from build123d import *

# Parameters (mm, degrees)
SKETCH1_R           = 381
SKETCH1_R_2         = 279.4
BOSS_EXTRUDE1_DEPTH = 19.05
CIRPATTERN1_COUNT   = 24


with BuildPart() as part:
    # Sketch1 → Boss-Extrude1 (new body)
    with BuildSketch(Plane(origin=(0, 0, 0), x_dir=(1, 0, 0), z_dir=(0, 1, 0))):
        Circle(SKETCH1_R)
        Circle(SKETCH1_R_2, mode=Mode.SUBTRACT)
    extrude(amount=BOSS_EXTRUDE1_DEPTH)

    # Sketch2 → 1 (1) Diameter Hole1 (revolve, cut)
    with BuildSketch(Plane(origin=(0, 19.05, -330.2), x_dir=(0, 0, 1), z_dir=(1, 0, 0))):
        Polygon((0, 0), (0, 39.630929862), (12.7, 32), (12.7, 0), align=None)
    f_1_1_diameter_hole1 = revolve(axis=Axis((0, 25.4, -330.2), (0, -1, 0)), mode=Mode.SUBTRACT)

    # CirPattern1: 1 (1) Diameter Hole1 ×24 about axis
    cirpattern1_axis = Axis((0, 0, 0), (0, 1, 0))
    for i in range(1, CIRPATTERN1_COUNT):
        add(f_1_1_diameter_hole1.rotate(cirpattern1_axis, i * 360 / CIRPATTERN1_COUNT), mode=Mode.SUBTRACT)


solid = part.part
Could you check a few things on this model? Use its own coordinates, in mm. Give positions to 0.01 mm unless a question says otherwise; leave off trailing zeros. Order: outer loops, then holes, each group sorted by start corner. A loop starts at its lowest first (then second) coordinate and runs counter-clockwise, first axis right, second up. Notation, with made-up numbers: (-11, 4) -> (10, 4) arc R21 cw to (10, 17) -> close; hole circle Ø7 at (70.5, 35.25). An arc over 180 degrees is marked (long way). Answer in a Markdown table with one row per item. Add a question column.
Item 1: We'd pull the mould along Z, two halves only. Please class faces 1 (the cylindrical face through (-302.35, 9.39, 231.83)), 2 (the flat face through (-115, 0, -256)), 3 (the cylindrical face through (273.37, 9.66, 163.45)): pulls with the +Z half, pulls with the -Z half, needs draft (parallel to the pull), parting line crosses it, or undercut.
Item 2: Imagine slicing it at C-C (y = 5.75). Count the separate pieces of the cut face and the enclosed holes in it, and give its area (3 significant figures).
Item 3: Imagine slicing it at A-A (z = -121.5). List the corners of the cut face in (x, y) for me, and give its area (3 significant figures).
Item 4: I'm going to push flat-ended pins straight in: P1, Ø6, axis at x = 59.5, y = 15.5, coming from the +Z side; P2, Ø2, axis at y = 13.5, z = 23.5, coming from the -X side; P3, Ø2, axis at y = 9.5, z = -265.5, coming from the +X side. Where does each tip first touch, or does it pass through?
Item 5: Please list where these lines run through material, in increasing order: probe 1 along Z at (x, y) = (0, 6.75); probe 2 along X at (y, z) = (6.5, 165.1); probe 3 along Z at (x, y) = (288, 9).
Item 6: Imagine slicing it at B-B (x = -43). List the corners of the cut face in (y, z) for me, and give its area (3 significant figures).
Result:
| question | item | result |
|---|---|---|
| 1 | face 1 | parting line crosses it |
| 1 | face 2 | needs draft |
| 1 | face 3 | undercut |
| 2 | separate pieces | 1 |
| 2 | enclosed holes | 25 |
| 2 | area | 199,000 mm2 |
| 3 | outline | (-361.11, 0) -> (-251.6, 0) -> (-251.6, 19.05) -> (-361.11, 19.05) -> close; (251.6, 0) -> (361.11, 0) -> (361.11, 19.05) -> (251.6, 19.05) -> close |
| 3 | area | 4,170 mm2 |
| 4 | P1 | z = 376.79 |
| 4 | P2 | x = -380.34 |
| 4 | P3 | x = 274.23 |
| 5 | probe 1 | -381 to -342.9, -317.5 to -279.4, 279.4 to 317.5, 342.9 to 381 |
| 5 | probe 2 | -343.37 to -298.66, -273.26 to -225.4, 225.4 to 273.26, 298.66 to 343.37 |
| 5 | probe 3 | -249.43 to -177.64, -152.56 to 152.56, 177.64 to 249.43 |
| 6 | outline | (0, -378.57) -> (19.05, -378.57) -> (19.05, -276.07) -> (0, -276.07) -> close; (0, 276.07) -> (19.05, 276.07) -> (19.05, 378.57) -> (0, 378.57) -> close |
| 6 | area | 3,910 mm2 |
